Verification items for the finished model (mm, model axes). Give positions to 0.01 mm unless a question says otherwise; leave off trailing zeros. Write each loop counter-clockwise with the first axis right and the second up, starting at its lowest first coordinate (ties: lowest second). Pieces come first, ordered by that corner, then holes. Notation, with made-up numbers: (-37, 29.25) - (-5, 29.25) arc R21 ccw to (-5, 57.25) - close; hole circle Ø4 at (-0.75, 9). An arc over 180 degrees is marked (long way). Put each result on its own line as item: value.
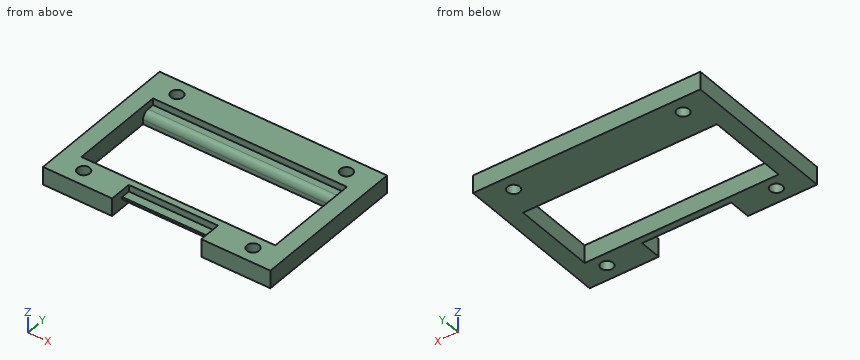
from build123d import *

# Parameters (mm, degrees)
SKETCH_W     = 87
SKETCH_H     = 37
PAD_DEPTH    = 5
SKETCH001_W  = 87
SKETCH001_H  = 43
PAD001_DEPTH = 3
CHAMFER_SIZE = 4
FILLET_R     = 3
SKETCH002_R  = 2.75
POCKET_DEPTH = 8.001


with BuildPart() as part:
    # Sketch → Pad (new body)
    with BuildSketch(Plane.XY):
        Polygon((-51, -31.5), (-51, 38.5), (51, 38.5), (51, -31.5), (20, -31.5), (20, -25.5), (-20, -25.5), (-20, -31.5), align=None)
        Rectangle(SKETCH_W, SKETCH_H, mode=Mode.SUBTRACT)
    extrude(amount=PAD_DEPTH)

    # Sketch001 (on Face14 of Pad) → Pad001 (join)
    with BuildSketch(Plane.XY.offset(5)):
        Polygon((-51, 38.5), (51, 38.5), (51, -31.5), (20, -31.5), (20, -21.5), (-20, -21.5), (-20, -31.5), (-51, -31.5), align=None)
        with Locations((0, 3)):
            Rectangle(SKETCH001_W, SKETCH001_H, mode=Mode.SUBTRACT)
    extrude(amount=PAD001_DEPTH)

    # Chamfer
    chamfer_edges = [part.edges().sort_by_distance(p)[0] for p in [
        (0, -25.5, 0),
    ]]
    chamfer(chamfer_edges, length=CHAMFER_SIZE)

    # Fillet
    fillet_edges = [part.edges().sort_by_distance(p)[0] for p in [
        (0, 18.5, 5),
    ]]
    fillet(fillet_edges, radius=FILLET_R)

    # Sketch002 (on Face18 of Fillet) → Pocket (cut, through all)
    with BuildSketch(Plane.XY.offset(8)):
        with Locations((-38, 31.5)):
            Circle(SKETCH002_R)
        with Locations((38, 31.5)):
            Circle(SKETCH002_R)
        with Locations((38, -24.5)):
            Circle(SKETCH002_R)
        with Locations((-38, -24.5)):
            Circle(SKETCH002_R)
    extrude(amount=-POCKET_DEPTH, mode=Mode.SUBTRACT)


solid = part.part
Q1. Section check B-B, the plane x = 10. Record the cut outline in (y, z).
Answers follow:
outline: (-25.5, 4) - (-21.5, 0) - (-18.5, 0) - (-18.5, 8) - (-21.5, 8) - (-21.5, 5) - (-25.5, 5) - close; (18.5, 0) - (38.5, 0) - (38.5, 8) - (24.5, 8) - (24.5, 5) - (21.5, 5) arc R3 ccw to (18.5, 2) - close
Q2. Section check A-A, the plane y = 31.5. Record the cut outline in (x, z).
Answers follow:
outline: (-51, 0) - (-40.75, 0) - (-40.75, 8) - (-51, 8) - close; (-35.25, 0) - (35.25, 0) - (35.25, 8) - (-35.25, 8) - close; (40.75, 0) - (51, 0) - (51, 8) - (40.75, 8) - close
Q3. Section check C-C, the plane y = 8. Record the cut outline in (x, z).
Answers follow:
outline: (-51, 0) - (-43.5, 0) - (-43.5, 8) - (-51, 8) - close; (43.5, 0) - (51, 0) - (51, 8) - (43.5, 8) - close
Q4. Go/stop test with flat-tipped pins: pin 1 Ø7 at (x, y) = (38, 31.5) entering from +Z; pin 2 Ø5 at (x, y) = (-38, -24.5) entering from -Z; pin 3 Ø0.8 at (x, z) = (9.5, 4.5) entering from -Y; pin 4 Ø0.9 at (x, z) = (18, 6) entering from -Y. Record where each tip stops, or that it passes through.
Answers follow:
pin 1: stops at z = 8
pin 2: passes through
pin 3: stops at y = -25.5
pin 4: stops at y = -21.5
Q5. Section check D-D, the plane z = 6.5. Record the cut outline in (x, y), plus the area to 3 significant figures.
Answers follow:
outline: (-51, -31.5) - (-20, -31.5) - (-20, -21.5) - (20, -21.5) - (20, -31.5) - (51, -31.5) - (51, 38.5) - (-51, 38.5) - close; hole (-43.5, -18.5) - (43.5, -18.5) - (43.5, 24.5) - (-43.5, 24.5) - close; hole circle Ø5.5 at (-38, -24.5); hole circle Ø5.5 at (-38, 31.5); hole circle Ø5.5 at (38, -24.5); hole circle Ø5.5 at (38, 31.5)
area: 2,900 mm2
Q6. Scan lines: line 1 along Y through (x, z) = (38, 5.5); line 2 along Y through (x, z) = (12, 5.5); line 3 along Y through (x, z) = (22, 6.75). Record each from-to range of solid material in increasing order.
Answers follow:
line 1: y = -31.5 to -27.25, -21.75 to -18.5, 24.5 to 28.75, 34.25 to 38.5
line 2: y = -21.5 to -18.5, 24.5 to 38.5
line 3: y = -31.5 to -18.5, 24.5 to 38.5
